Answer from the drawing. Dimensions are ordinates in mm from the lowest x, y and z of the part. Give positions to 0.01 mm unless a question says otherwise; leave off trailing zeros. Write each loop counter-clockwise with the first axis right and the second up, starting at its lowest first coordinate (ties: lowest second). Pieces come first, ordered by that corner, then holes. Notation, with made-up numbers: (63, 14) - (107, 14) arc R17 ccw to (107, 38) - close; hole circle Ø7 at (-13.5, 83.5). An arc over 180 degrees is marked (long way). Write item = value, one per line.
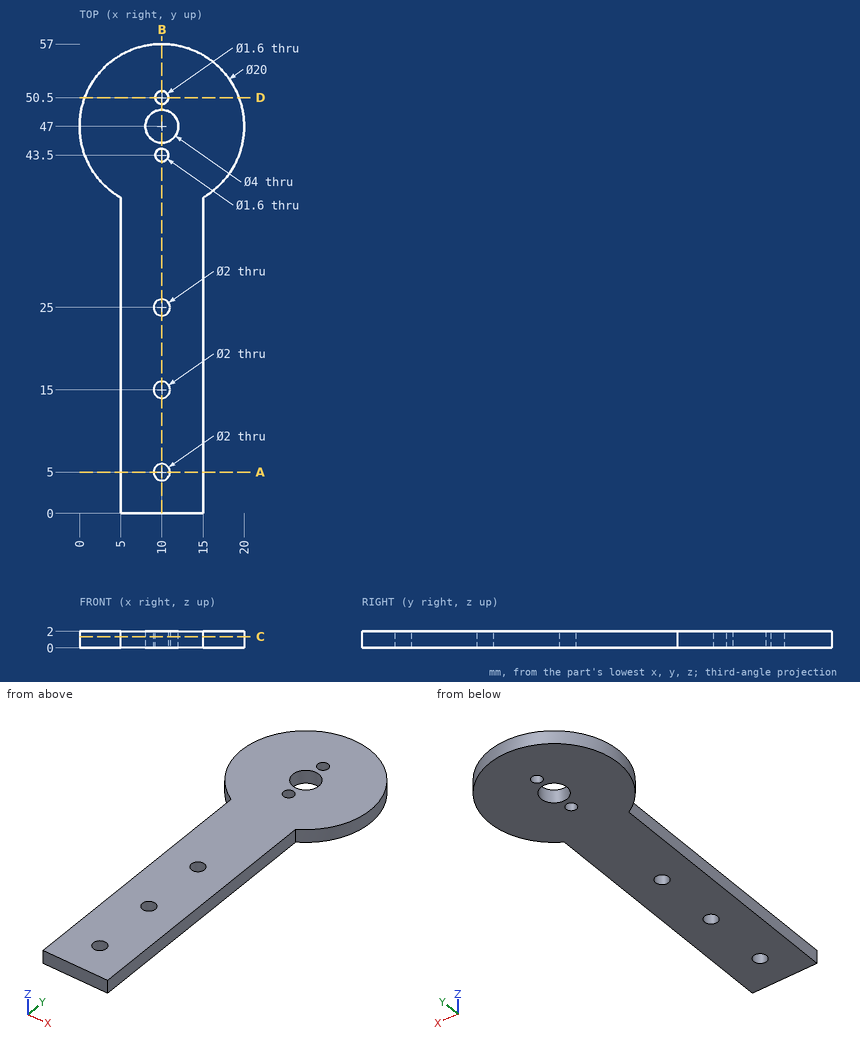
1. Given pin 1 (1.8 mm diameter, centred on x = 10, y = 43.5, fed in from -Z); pin 2 (1.6 mm diameter, centred on x = 10, y = 15, fed in from -Z); pin 3 (0.6 mm diameter, centred on y = 23.5, z = 1.5, fed in from -X); pin 4 (0.6 mm diameter, centred on y = 20.5, z = 1.5, fed in from +X), each flat-ended and moving along its own axis, determine where each tip first touches the part or whether it passes through.
Solution:
pin_1 = 0
pin_2 = through
pin_3 = 5
pin_4 = 15
2. Find section D-D, the plane y = 50.5. Give the vertices of the cut face in (x, z), then the cut area to 3 significant figures.
Solution:
outline = (0.63, 0) - (9.2, 0) - (9.2, 2) - (0.63, 2) - close; (10.8, 0) - (19.37, 0) - (19.37, 2) - (10.8, 2) - close
area = 34.3 mm^2
3. Find section B-B, the plane x = 10. Give the vertices of the cut face in (y, z).
Solution:
outline = (0, 0) - (4, 0) - (4, 2) - (0, 2) - close; (6, 0) - (14, 0) - (14, 2) - (6, 2) - close; (16, 0) - (24, 0) - (24, 2) - (16, 2) - close; (26, 0) - (42.7, 0) - (42.7, 2) - (26, 2) - close; (44.3, 0) - (45, 0) - (45, 2) - (44.3, 2) - close; (49, 0) - (49.7, 0) - (49.7, 2) - (49, 2) - close; (51.3, 0) - (57, 0) - (57, 2) - (51.3, 2) - close
4. Find section C-C, the plane z = 1.35. Give the vertices of the cut face in (x, y).
Solution:
outline = (5, 0) - (15, 0) - (15, 38.34) arc R10 ccw (long way) to (5, 38.34) - close; hole circle Ø4 at (10, 47); hole circle Ø2 at (10, 5); hole circle Ø2 at (10, 15); hole circle Ø2 at (10, 25); hole circle Ø1.6 at (10, 43.5); hole circle Ø1.6 at (10, 50.5)
5. Straight lines are drawn through the part: line 1 (X direction, y = 51, z = 1.1); line 2 (X direction, y = 46, z = 0.4); line 3 (X direction, y = 33, z = 0.7). For each, find the intervals that lie inside material, in ascending order.
Solution:
line_1 = 0.83 to 9.38, 10.62 to 19.17
line_2 = 0.05 to 8.27, 11.73 to 19.95
line_3 = 5 to 15
6. Find section A-A, the plane y = 5. Give the vertices of the cut face in (x, z), then the cut area to 3 significant figures.
Solution:
outline = (5, 0) - (9, 0) - (9, 2) - (5, 2) - close; (11, 0) - (15, 0) - (15, 2) - (11, 2) - close
area = 16.0 mm^2
